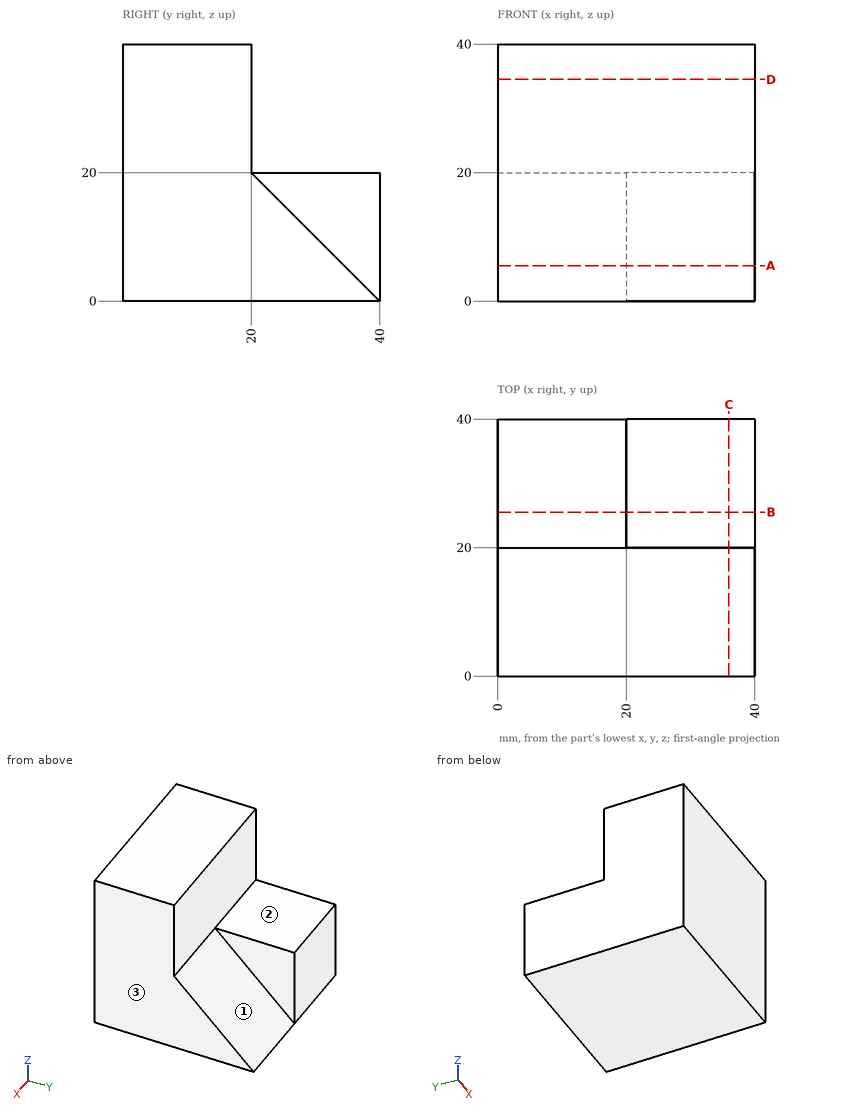
Job drawing, mm, ordinate dimensions from the low corner. One solid piece. A direction names the side the tool comes from. Round coordinates to 2 decimals unless told otherwise and drop trailing zeros. Loops run counter-clockwise (first coordinate to the right, second up) from the corner with the lowest first, then second, coordinate; pieces in that order, holes last.
(1) Cut at A-A (z = 5.5). Give the cut face in (x, y), plus the area to 3 significant figures.
(2) Which spindle directions (+Z, -Z, +X, -X, +Y, -Y) get a long thin tool onto all of the face, cutting with end or side? Do the marked faces 1, 2 and 3. Say none if no direction does.
(3) Cut at C-C (x = 36). Give the cut face in (y, z).
(4) Wall check: line 1 along Y through (x, z) = (22, 29.5). Give the ranges that are in metal, low to high.
(5) Cut at B-B (y = 25.5). Give the cut face in (x, z), plus the area to 3 significant figures.
(6) Cut at D-D (z = 34.5). Give the cut face in (x, y), plus the area to 3 significant figures.
(7) Drop flat-ended pins along their axis: pin 1 (1 mm diameter, centred on x = 26, z = 29.5, fed in from +Y); pin 2 (1.5 mm diameter, centred on x = 30, z = 7.5, fed in from +Y); pin 3 (6 mm diameter, centred on y = 29.5, z = 17.5, fed in from +X). Give the stop position or say it passes through.
Findings below:
1. outline: (0, 0) - (40, 0) - (40, 34.5) - (20, 34.5) - (20, 40) - (0, 40) - close
1. area: 1,490 mm2
2. face 1: +Z, +X, +Y
2. face 2: +Z, +X, -X, +Y
2. face 3: +Z, -Z, +X, +Y, -Y
3. outline: (0, 0) - (40, 0) - (20, 20) - (20, 40) - (0, 40) - close
4. line 1: y = 0 to 20
5. outline: (0, 0) - (40, 0) - (40, 14.5) - (20, 14.5) - (20, 20) - (0, 20) - close
5. area: 690 mm2
6. outline: (0, 0) - (40, 0) - (40, 20) - (0, 20) - close
6. area: 800 mm2
7. pin 1: stops at y = 20
7. pin 2: stops at y = 33.25
7. pin 3: stops at x = 20
